from build123d import *

# Parameters (mm, degrees)
SKETCH1_W           = 48
SKETCH1_H           = 84
BOSS_EXTRUDE1_DEPTH = 4.5
FILLET1_R           = 2
CUT_EXTRUDE1_DEPTH  = 49.582404222
BOSS_EXTRUDE2_DEPTH = 48.5
RIB1_REACH          = 104.181
SKETCH4_WALL_W      = 252.541422716
SKETCH4_WALL_H      = 3
RIB14_REACH         = 80.032
SKETCH5_WALL_W      = 204.243088956
SKETCH5_WALL_H      = 3
SKETCH6_R           = 11.1
CUT_EXTRUDE2_DEPTH  = 8
SKETCH7_W           = 14
SKETCH7_H           = 15
BOSS_EXTRUDE3_DEPTH = 20
FILLET2_R           = 7
FILLET3_R           = 2
SKETCH8_R           = 4
CUT_EXTRUDE3_DEPTH  = 10
CUT_EXTRUDE4_DEPTH  = 69.5


with BuildPart() as part:
    # Sketch1 → Boss-Extrude1 (new body)
    with BuildSketch(Plane(origin=(0, 0, 0), x_dir=(1, 0, 0), z_dir=(0, 1, 0))):
        Rectangle(SKETCH1_W, SKETCH1_H)
    extrude(amount=BOSS_EXTRUDE1_DEPTH)

    # Fillet1
    fillet1_edges = [part.edges().sort_by_distance(p)[0] for p in [
        (-24, 2.25, -42),
        (24, 2.25, -42),
        (24, 2.25, 42),
        (-24, 2.25, 42),
    ]]
    fillet(fillet1_edges, radius=FILLET1_R)

    # Sketch2 → Cut-Extrude1 (cut, through all)
    with BuildSketch(Plane(origin=(0, 4.5, 0), x_dir=(1, 0, 0), z_dir=(0, 1, 0))):
        with BuildLine():
            Line((-5.25, 33.5), (13.25, 33.5))
            ThreePointArc((13.25, 33.5), (16, 30.750000115), (13.25000023, 28))
            Line((13.25000023, 28), (-5.25, 28))
            ThreePointArc((-5.25, 28), (-8, 30.75), (-5.25, 33.5))
        make_face()
        with BuildLine():
            Line((-5.25, 3), (13.25000023, 3))
            ThreePointArc((13.25000023, 3), (16, 0.249999885), (13.25, -2.5))
            Line((13.25, -2.5), (-5.25, -2.5))
            ThreePointArc((-5.25, -2.5), (-8, 0.25), (-5.25, 3))
        make_face()
    extrude(amount=-CUT_EXTRUDE1_DEPTH, mode=Mode.SUBTRACT)

    # Sketch3 → Boss-Extrude2 (add)
    with BuildSketch(Plane(origin=(0, 4.5, 0), x_dir=(1, 0, 0), z_dir=(0, 1, 0))):
        with BuildLine():
            Line((-11.5, 42), (-22, 42))
            ThreePointArc((-22, 42), (-23.414213562, 41.414213562), (-24, 40))
            Line((-24, 40), (-24, -10))
            Line((-24, -10), (-11.5, -10))
            Line((-11.5, -10), (-11.5, 42))
        make_face()
    extrude(amount=BOSS_EXTRUDE2_DEPTH)

    # Sketch4 wall → Rib1 (add, up to next)
    with BuildSketch(Plane(origin=(1.25, 23.75, -42), x_dir=(-0.552199056825, 0.833712301481, 0), z_dir=(0.833712301481, 0.552199056825, 0)), mode=Mode.PRIVATE) as rib1_sk1:
        with Locations((0, 1.5)):
            Rectangle(SKETCH4_WALL_W, SKETCH4_WALL_H)
    rib1_tool1 = extrude(rib1_sk1.sketch, amount=-RIB1_REACH, mode=Mode.PRIVATE) - part.part
    add(rib1_tool1.solids().sort_by_distance((1.25, 23.75, -42))[0])

    # Sketch5 wall → Rib14 (add, up to next)
    with BuildSketch(Plane(origin=(1.25, 23.75, 10), x_dir=(-0.552199056825, 0.833712301481, 0), z_dir=(-0.833712301481, -0.552199056825, 0)), mode=Mode.PRIVATE) as rib14_sk1:
        with Locations((0, 1.5)):
            Rectangle(SKETCH5_WALL_W, SKETCH5_WALL_H)
    rib14_tool1 = extrude(rib14_sk1.sketch, amount=RIB14_REACH, mode=Mode.PRIVATE) - part.part
    add(rib14_tool1.solids().sort_by_distance((1.25, 23.75, 10))[0])

    # Sketch6 → Cut-Extrude2 (cut)
    with BuildSketch(Plane.ZY.offset(24)):
        with Locations((-16, 25.65)):
            Circle(SKETCH6_R)
    extrude(amount=-CUT_EXTRUDE2_DEPTH, mode=Mode.SUBTRACT)

    # Sketch7 → Boss-Extrude3 (add)
    with BuildSketch(Plane(origin=(0, 4.5, 0), x_dir=(1, 0, 0), z_dir=(0, 1, 0))):
        with Locations((-10, -27)):
            Rectangle(SKETCH7_W, SKETCH7_H)
    extrude(amount=BOSS_EXTRUDE3_DEPTH)

    # Fillet2
    fillet2_edges = [part.edges().sort_by_distance(p)[0] for p in [
        (-10, 4.5, 34.5),
        (-10, 4.5, 19.5),
    ]]
    fillet(fillet2_edges, radius=FILLET2_R)

    # Fillet3
    fillet3_edges = [part.edges().sort_by_distance(p)[0] for p in [
        (-10, 24.5, 34.5),
        (-10, 24.5, 19.5),
    ]]
    fillet(fillet3_edges, radius=FILLET3_R)

    # Sketch8 → Cut-Extrude3 (cut)
    with BuildSketch(Plane.ZY.offset(17)):
        with Locations((27, 16.5)):
            Circle(SKETCH8_R)
    extrude(amount=-CUT_EXTRUDE3_DEPTH, mode=Mode.SUBTRACT)

    # Sketch9 → Cut-Extrude4 (cut, through all)
    with BuildSketch(Plane(origin=(0, 4.5, 0), x_dir=(1, 0, 0), z_dir=(0, 1, 0))):
        with BuildLine():
            Line((2.75, -24.25), (15.25, -24.25))
            ThreePointArc((15.25, -24.25), (18, -27), (15.25, -29.75))
            Line((15.25, -29.75), (2.75, -29.75))
            ThreePointArc((2.75, -29.75), (0, -27), (2.75, -24.25))
        make_face()
    extrude(amount=-CUT_EXTRUDE4_DEPTH, mode=Mode.SUBTRACT)


solid = part.part
Work out the finished part from the listing and answer in its coordinate system (mm). A direction names the side the tool comes from. Coordinates: 2 decimals unless noted, no trailing zeros. Write each loop counter-clockwise with the first axis right and the second up, starting at its lowest first coordinate (ties: lowest second). Pieces come first, ordered by that corner, then holes. Notation, with made-up numbers: M 29,3 L 67,3 A15 ccw 67,17 Z; hole C 70.25,77.5 d5. An arc over 180 degrees is marked long. Use one line per item in the form item = value. Start each with the question number.
1. The part is cut by section D-D (y = 38.5). Give the vertices of the cut face in (x, z).
2. The part is cut by section C-C (x = -10). Give the vertices of the cut face in (y, z), plus the area to 3 significant figures.
3. Each of these flat-tipped pins is pushed along its axis until it touches: P1, Ø6, axis at y = 18.5, z = 25.5, coming from the -X side; P2, Ø10.5, axis at y = 16.5, z = 27, coming from the +X side; P3, Ø2, axis at y = 18, z = -20, coming from the +X side; P4, Ø7.5, axis at x = 7, y = 23.5, coming from the -Z side. Where does it stop, or does it pass through?
4. Straight lines are drawn through the part: probe 1 along Y at (x, z) = (-18.5, -16); probe 2 along Y at (x, z) = (-11, 27); probe 3 along Z at (x, y) = (-10, 16). For each, find the intervals that lie inside material, in ascending order. Write a range as from..to.
5. The part is cut by section A-A (z = 27). Give the vertices of the cut face in (x, y), plus the area to 3 significant figures.
6. A tool of negligible diameter and unlimited length cuts with its end or side. For faces 1 (the face through (-7, 17, 27)), 2 (the face through (4, 2, -28)), 3 (the face through (-5, 19, 7)), 4 (the face through (-10, 25, 10)), 5 (the face through (-17, 12, 27)), from which of +Z, -Z, +X, -X, +Y, -Y can it reach the whole face along a straight path? Write none if from no direction.
7. The part is cut by section B-B (x = 11). Give the vertices of the cut face in (y, z), plus the area to 3 significant figures.
8. The mould has two halves that part along Z. Classify faces 6 (the face through (4, 2, -33.5)), 7 (the face through (18, 2, 27)), 8 (the face through (-24, 14, -9)), 9 (the face through (-23.4, 26.13, -41.43)): released by +Z, released by -Z, zero draft, split by the parting line, or undercut.
Evaluation:
q1.outline = M -24,-40 A2 ccw -22,-42 L -8.52,-42 L -8.52,-39 L -11.5,-39 L -11.5,7 L -8.52,7 L -8.52,10 L -24,10 Z
q2.outline = M 0,-42 L 40.74,-42 L 40.74,-39 L 4.5,-39 L 4.5,7 L 40.74,7 L 40.74,10 L 4.5,10 L 4.5,12.5 A7 cw 11.5,19.5 L 22.5,19.5 A2 ccw 24.5,21.5 L 24.5,32.5 A2 ccw 22.5,34.5 L 11.5,34.5 A7 cw 4.5,41.5 L 4.5,42 L 0,42 Z; hole C 16.5,27 d8
q2.area = 864 mm^2
q3.P1 = -17
q3.P2 = -3
q3.P3 = -11.5
q3.P4 = through
q4.probe_1 = 0..14.55, 36.75..53
q4.probe_2 = 0..12.5, 20.5..24.5
q4.probe_3 = -42..-39, 7..10, 19.5..23.03, 30.97..34.5
q5.outline = M -24,0 L 0,0 L 0,4.5 L -3,4.5 L -3,24.5 L -17,24.5 L -17,20.5 L -7,20.5 L -7,12.5 L -17,12.5 L -17,4.5 L -24,4.5 Z; M 18,0 L 24,0 L 24,4.5 L 18,4.5 Z
q5.area = 335 mm^2
q6.face_1 = -X
q6.face_2 = +Y, -Y
q6.face_3 = +X, +Y
q6.face_4 = +X, -X, +Y
q6.face_5 = +Z, -X, +Y
q7.outline = M 0,-42 L 9.03,-42 L 9.03,-39 L 4.5,-39 L 4.5,-33.5 L 0,-33.5 Z; M 0,-28 L 4.5,-28 L 4.5,-3 L 0,-3 Z; M 0,2.5 L 4.5,2.5 L 4.5,7 L 9.03,7 L 9.03,10 L 4.5,10 L 4.5,24.25 L 0,24.25 Z; M 0,29.75 L 4.5,29.75 L 4.5,42 L 0,42 Z
q7.area = 331 mm^2
q8.face_6 = undercut
q8.face_7 = undercut
q8.face_8 = zero draft
q8.face_9 = released by -Z
